```python
from build123d import *

# Parameters (mm, degrees)
F1_DEPTH = 38.1
F3_DEPTH = 19.05
F4_R     = 6.6122304169
F5_DEPTH = 254


with BuildPart() as f1:
    # F0 (on Front) → F1 (new body, symmetric)
    with BuildSketch(Plane.XZ):
        Polygon((0, -33.1354551017), (75.9690925479, -33.1354551017), (0, 33.1354551017), (-75.9690925479, 33.1354551017), (-75.9690925479, -20.4354561865), (0, -20.4354561865), align=None)
    extrude(amount=F1_DEPTH, both=True)

    # F2 (on face) → F3 (cut)
    with BuildSketch(Plane.XZ.offset(38.1)):
        Polygon((22.7042404154, -33.1354551017), (75.9690925479, -33.1354551017), (22.7042404154, 13.3296284511), align=None)
    extrude(amount=-F3_DEPTH, mode=Mode.SUBTRACT)

    # F4 (on face) → F5 (cut)
    with BuildSketch(Plane(origin=(-75.9690925479, 0, 0), x_dir=(0, -1, 0), z_dir=(-1, 0, 0))):
        with Locations((7.1581806988, 20.4354561865)):
            Circle(F4_R)
        with Locations((-20.0890917331, -4.0409089997)):
            Circle(F4_R)
        with Locations((7.1581806988, -4.0409089997)):
            Circle(F4_R)
        with Locations((-20.0890917331, 20.4354561865)):
            Circle(F4_R)
    extrude(amount=-F5_DEPTH, mode=Mode.SUBTRACT)


solid = f1.part
```
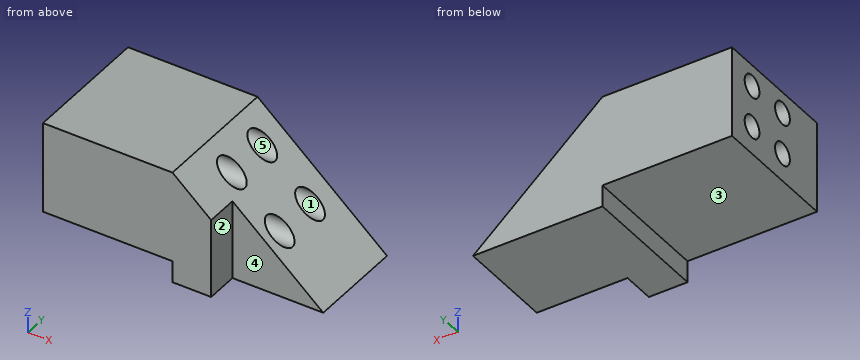
Can you work these out from the model? Positions are in its coordinate system, mm. Face numbers are marked on the shaded views. A direction names the side the tool comes from. Coordinates: 2 decimals unless noted, no trailing zeros. Loops run counter-clockwise (first coordinate to the right, second up) from the corner with the lowest first, then second, coordinate; pieces in that order, holes last. Notation, with made-up numbers: (52, 46.25) -> (82, 46.25) arc R24 cw to (82, 58.25) -> close; hole circle Ø3 at (5, -22). An arc over 180 degrees is marked (long way). Put each result on its own line as item: value. Start each with the question number.
Q1. Thinking about a two-plate mould opening in Y: for the marked faces 3, 4 and 5, which applies, pulls with the +Y half, pulls with the -Y half, needs draft (parallel to the pull), parting line crosses it, or undercut?
Q2. I'm going to push flat-ended pins straight in: P1, Ø6, axis at x = 23, y = 9.5, coming from the +Z side; P2, Ø8, axis at x = -21.5, y = 1.5, coming from the -Z side; P3, Ø9.5, axis at y = -27, z = -4.5, coming from the +X side. Where does each tip first touch, or does it pass through?
Q3. If I drill on line 1 (Z direction, x = 15, y = 20.5); line 2 (Y direction, x = -39.5, z = -2); line 3 (Z direction, x = -0.5, y = -2), over which ranges is the centre line in solid material (lowest first)? Write a range as [from, to].
Q4. For the marked faces 1 and 2, which set-ups out of +Z, -Z, +X, -X, +Y, -Y let a thin tool reach every point of the face, with its end or its side?
Q5. I want a section at D-D (y = -17.5). Write out the boundary of the cut face in (x, z).
Q6. I want a section at C-C (x = 3). Write out the boundary of the cut face in (y, z).
Q7. I want a section at A-A (z = 22.5). Write out the boundary of the cut face in (x, y).
Q8. I want a section at B-B (y = 23). Write out the boundary of the cut face in (x, z).
Taken from the geometry:
1. face 3: needs draft
1. face 4: pulls with the -Y half
1. face 5: undercut
2. P1: stops at z = 15.69
2. P2: stops at z = -20.44
2. P3: stops at x = 22.7
3. line 1: z = [-33.14, -10.64], [2.56, 13.84]
3. line 2: y = [-38.1, -13.45], [-0.87, 13.8], [26.38, 38.1]
3. line 3: z = [-20.44, -8.18], [0.1, 16.3], [24.57, 33.14]
4. face 1: +X, -X
4. face 2: +Z, -Z, +X, -Y
5. outline: (-75.97, -20.44) -> (0, -20.44) -> (0, -33.14) -> (75.97, -33.14) -> (0, 33.14) -> (-75.97, 33.14) -> close
6. outline: (-38.1, -33.14) -> (38.1, -33.14) -> (38.1, 30.52) -> (-38.1, 30.52) -> close; hole circle Ø13.22 at (-7.16, -4.04); hole circle Ø13.22 at (-7.16, 20.44); hole circle Ø13.22 at (20.09, -4.04); hole circle Ø13.22 at (20.09, 20.44)
7. outline: (-75.97, -38.1) -> (12.19, -38.1) -> (12.19, -13.44) -> (-75.97, -13.44) -> close; (-75.97, -0.88) -> (12.19, -0.88) -> (12.19, 13.81) -> (-75.97, 13.81) -> close; (-75.97, 26.37) -> (12.19, 26.37) -> (12.19, 38.1) -> (-75.97, 38.1) -> close
8. outline: (-75.97, -20.44) -> (0, -20.44) -> (0, -33.14) -> (75.97, -33.14) -> (49.42, -9.98) -> (-75.97, -9.98) -> close; (-75.97, 1.9) -> (35.81, 1.9) -> (21.36, 14.5) -> (-75.97, 14.5) -> close; (-75.97, 26.37) -> (7.75, 26.37) -> (0, 33.14) -> (-75.97, 33.14) -> close
